Build history of the part. All positions in model axes, mm. Coordinates: 2 decimals unless noted, no trailing zeros. Order: outer loops, then holes, each group sorted by start corner. A loop starts at its lowest first (then second) coordinate and runs counter-clockwise, first axis right, second up. Notation, with made-up numbers: (-21.5, -8.5) - (15.5, -8.5) arc R27 cw to (15.5, 12.5) - close; hole circle Ø5 at (18, 83). An arc over 180 degrees is marked (long way). Write each question's results on one line, items separated by ' | '. Start each with the question number.
from build123d import *

# Parameters (mm, degrees)
SKETCH1_W                     = 200
SKETCH1_H                     = 80
BOSS_EXTRUDE1_DEPTH           = 10
CSK_FOR_M8_SFHCS1_D           = 8.4
CSK_FOR_M8_SFHCS1_CSINK_D     = 17.92
CSK_FOR_M8_SFHCS1_CSINK_ANGLE = 90
M4_CLEARANCE_HOLE1_D          = 4.5
FILLET1_R                     = 10


with BuildPart() as part:
    # Sketch1 → Boss-Extrude1 (new body)
    with BuildSketch(Plane(origin=(0, 0, 0), x_dir=(1, 0, 0), z_dir=(0, 1, 0))):
        Rectangle(SKETCH1_W, SKETCH1_H)
    extrude(amount=BOSS_EXTRUDE1_DEPTH)

    # CSK for M8 SFHCS1 (through all)
    with Locations(Plane(origin=(0, 10, 0), x_dir=(1, 0, 0), z_dir=(0, 1, 0))):
        with Locations((-20, 20), (20, -20), (60, -20), (-20, -20), (-60, -20), (60, 20), (20, 20), (-60, 20)):
            CounterSinkHole(CSK_FOR_M8_SFHCS1_D / 2, CSK_FOR_M8_SFHCS1_CSINK_D / 2, counter_sink_angle=CSK_FOR_M8_SFHCS1_CSINK_ANGLE)

    # M4 Clearance Hole1 (through all)
    with Locations(Plane(origin=(0, 10, 0), x_dir=(1, 0, 0), z_dir=(0, 1, 0))):
        with Locations((-90, 20), (90, 20), (90, -20), (-90, -20)):
            Hole(M4_CLEARANCE_HOLE1_D / 2)

    # Fillet1
    fillet1_edges = [part.edges().sort_by_distance(p)[0] for p in [
        (100, 5, 40),
        (-100, 5, 40),
        (-100, 5, -40),
        (100, 5, -40),
    ]]
    fillet(fillet1_edges, radius=FILLET1_R)


solid = part.part
Item 1: Probe probe 1 along Z at (x, y) = (90, 6); probe 2 along Z at (x, y) = (20, 1.6); probe 3 along X at (y, z) = (7, -31). List the from-to ranges inside material, lowest first.
Item 2: Slice it at B-B (y = 7.75). Count the separate pieces of the cut face and the enclosed holes in it, then the cut area to 3 significant figures.
Item 3: Slice it at A-A (x = -60). Write the cut outline in (y, z).
Item 4: Flat gauge pins, fed straight in: P1, Ø6, axis at x = 90, z = 20, coming from the +Y side; P2, Ø9.5, axis at x = -20, z = 20, coming from the +Y side. Where does each tip first touch, or does it go through?
Item 5: Pull direction Z, two halves, no side cores. Call faces 1 (the cylindrical face through (-97.15, 5.07, 36.99)), 2 (the cylindrical face through (-55.804, 2.583, -20.185)), 3 (the cylindrical face through (-97.15, 5.07, -36.99)): released by +Z, released by -Z, zero draft, split by the parting line, or undercut.
Resolved:
1) probe 1: -40 to -22.25, -17.75 to 17.75, 22.25 to 40 | probe 2: -40 to -24.2, -15.8 to 15.8, 24.2 to 40 | probe 3: -99.95 to 99.95
2) separate pieces: 1 | enclosed holes: 12 | area: 14,700 mm^2
3) outline: (0, -40) - (10, -40) - (10, -28.96) - (5.24, -24.2) - (0, -24.2) - close; (0, -15.8) - (5.24, -15.8) - (10, -11.04) - (10, 11.04) - (5.24, 15.8) - (0, 15.8) - close; (0, 24.2) - (5.24, 24.2) - (10, 28.96) - (10, 40) - (0, 40) - close
4) P1: y = 10 | P2: y = 5.79
5) face 1: released by +Z | face 2: undercut | face 3: released by -Z
